from build123d import *

# Parameters (mm, degrees)
SKETCH1_R                    = 3
SKETCH1_R_2                  = 4
BASE_FLANGE1_DEPTH           = 2
SKETCH6_W                    = 90.588867986
SKETCH6_H                    = 42.612496281
CUT_EXTRUDE1_DEPTH           = 10
DELETEFACE2_START            = -2
DELETEFACE2_DEPTH            = 2
DELETEFACE3_START            = 50
DELETEFACE3_OUTLINE_W        = 40
DELETEFACE3_OUTLINE_H        = 2
DELETEFACE3_DEPTH            = 10
EDGE_FLANGE1_STRIP_W         = 9.4732
EDGE_FLANGE1_STRIP_H         = 2
EDGE_FLANGE1_STRIP_CUT_DEPTH = 40
EDGE_FLANGE1_DEPTH           = 40
EDGE_FLANGE2_STRIP_W         = 9.4732
EDGE_FLANGE2_STRIP_H         = 2
EDGE_FLANGE2_STRIP_CUT_DEPTH = 40
EDGE_FLANGE2_DEPTH           = 40
SKETCH15_R                   = 2.5
CUT_EXTRUDE2_DEPTH           = 10
CHAMFER1_SIZE                = 5
FILLET1_R                    = 5


# Read off the part's stored shape, not the designer's step: DeleteFace2, DeleteFace3
# Sheet-metal steps are written as plain solids
with BuildPart() as part:
    # Sketch1 → Base-Flange1 (new body)
    with BuildSketch(Plane(origin=(0, 0, 0), x_dir=(1, 0, 0), z_dir=(0, 1, 0))):
        with BuildLine():
            Line((-17.071067812, 52.928932188), (-12.928932188, 57.071067812))
            ThreePointArc((-12.928932188, 57.071067812), (-9.6846987, 59.238795325), (-5.857864376, 60))
            Line((-5.857864376, 60), (5.857864376, 60))
            ThreePointArc((5.857864376, 60), (9.6846987, 59.238795325), (12.928932188, 57.071067812))
            Line((12.928932188, 57.071067812), (17.071067812, 52.928932188))
            ThreePointArc((17.071067812, 52.928932188), (19.238795325, 49.6846987), (20, 45.857864376))
            Line((20, 45.857864376), (20, -45.857864376))
            ThreePointArc((20, -45.857864376), (19.238795325, -49.6846987), (17.071067812, -52.928932188))
            Line((17.071067812, -52.928932188), (12.928932188, -57.071067812))
            ThreePointArc((12.928932188, -57.071067812), (9.6846987, -59.238795325), (5.857864376, -60))
            Line((5.857864376, -60), (-5.857864376, -60))
            ThreePointArc((-5.857864376, -60), (-9.6846987, -59.238795325), (-12.928932188, -57.071067812))
            Line((-12.928932188, -57.071067812), (-17.071067812, -52.928932188))
            ThreePointArc((-17.071067812, -52.928932188), (-19.238795325, -49.6846987), (-20, -45.857864376))
            Line((-20, -45.857864376), (-20, -39.142135624))
            ThreePointArc((-20, -39.142135624), (-20.761204675, -35.3153013), (-22.928932188, -32.071067812))
            Line((-22.928932188, -32.071067812), (-27.071067812, -27.928932188))
            ThreePointArc((-27.071067812, -27.928932188), (-30.3153013, -25.761204675), (-34.142135624, -25))
            Line((-34.142135624, -25), (-45.857864376, -25))
            ThreePointArc((-45.857864376, -25), (-49.6846987, -24.238795325), (-52.928932188, -22.071067812))
            Line((-52.928932188, -22.071067812), (-57.071067812, -17.928932188))
            ThreePointArc((-57.071067812, -17.928932188), (-59.238795325, -14.6846987), (-60, -10.857864376))
            Line((-60, -10.857864376), (-60, 10.857864376))
            ThreePointArc((-60, 10.857864376), (-59.238795325, 14.6846987), (-57.071067812, 17.928932188))
            Line((-57.071067812, 17.928932188), (-52.928932188, 22.071067812))
            ThreePointArc((-52.928932188, 22.071067812), (-49.6846987, 24.238795325), (-45.857864376, 25))
            Line((-45.857864376, 25), (-34.142135624, 25))
            ThreePointArc((-34.142135624, 25), (-30.3153013, 25.761204675), (-27.071067812, 27.928932188))
            Line((-27.071067812, 27.928932188), (-22.928932188, 32.071067812))
            ThreePointArc((-22.928932188, 32.071067812), (-20.761204675, 35.3153013), (-20, 39.142135624))
            Line((-20, 39.142135624), (-20, 45.857864376))
            ThreePointArc((-20, 45.857864376), (-19.238795325, 49.6846987), (-17.071067812, 52.928932188))
        make_face()
        with Locations(Location((0, 42.5, 0), (0, 0, 270))):
            Circle(SKETCH1_R, mode=Mode.SUBTRACT)
        with Locations(Location((0, -42.5, 0), (0, 0, 270))):
            Circle(SKETCH1_R, mode=Mode.SUBTRACT)
        with Locations(Location((0, 0, 0), (0, 0, 270))):
            Circle(SKETCH1_R_2, mode=Mode.SUBTRACT)
        with Locations(Location((-35.23885867, -15, 0), (0, 0, 270))):
            Circle(SKETCH1_R_2, mode=Mode.SUBTRACT)
        with Locations(Location((-35.23885867, 15, 0), (0, 0, 270))):
            Circle(SKETCH1_R_2, mode=Mode.SUBTRACT)
    extrude(amount=-BASE_FLANGE1_DEPTH)

    # Sketch6 → Cut-Extrude1 (cut)
    with BuildSketch(Plane(origin=(0, 0, 0), x_dir=(1, 0, 0), z_dir=(0, 1, 0))):
        with Locations((11.152298369, 46.306248141)):
            Rectangle(SKETCH6_W, SKETCH6_H)
    extrude(amount=-CUT_EXTRUDE1_DEPTH, mode=Mode.SUBTRACT)

    # DeleteFace2 outline → DeleteFace2 (add)
    with BuildSketch(Plane(origin=(0, 0, 0), x_dir=(1, 0, 0), z_dir=(0, 1, 0)).offset(DELETEFACE2_START)):
        with BuildLine():
            Line((5.857864376, -60), (10, -60))
            Line((10, -60), (12.928932188, -57.071067812))
            ThreePointArc((12.928932188, -57.071067812), (9.6846987, -59.238795325), (5.857864376, -60))
        make_face()
        with BuildLine():
            Line((-20, -50), (-17.071067812, -52.928932188))
            ThreePointArc((-17.071067812, -52.928932188), (-19.238795325, -49.6846987), (-20, -45.857864376))
            Line((-20, -45.857864376), (-20, -50))
        make_face()
        with BuildLine():
            Line((-10, -60), (-5.857864376, -60))
            ThreePointArc((-5.857864376, -60), (-9.6846987, -59.238795325), (-12.928932188, -57.071067812))
            Line((-12.928932188, -57.071067812), (-10, -60))
        make_face()
        with BuildLine():
            ThreePointArc((20, -45.857864376), (19.238795325, -49.6846987), (17.071067812, -52.928932188))
            Line((17.071067812, -52.928932188), (20, -50))
            Line((20, -50), (20, -45.857864376))
        make_face()
    extrude(amount=DELETEFACE2_DEPTH)

    # DeleteFace3 outline → DeleteFace3 (add)
    with BuildSketch(Plane.XY.offset(DELETEFACE3_START)):
        with Locations((0, -1)):
            Rectangle(DELETEFACE3_OUTLINE_W, DELETEFACE3_OUTLINE_H)
    extrude(amount=DELETEFACE3_DEPTH)

    # Edge-Flange1 strip (across the edge) → Edge-Flange1 strip cut (cut)
    with BuildSketch(Plane(origin=(-20, 0, 60), x_dir=(0, 0, -1), z_dir=(1, 0, 0))):
        with Locations((-2, -1)):
            Rectangle(EDGE_FLANGE1_STRIP_W, EDGE_FLANGE1_STRIP_H)
    extrude(amount=EDGE_FLANGE1_STRIP_CUT_DEPTH, mode=Mode.SUBTRACT)

    # Edge-Flange1 section (across the edge) → Edge-Flange1 (add)
    with BuildSketch(Plane(origin=(-20, 0, 60), x_dir=(0, 0, -1), z_dir=(1, 0, 0))):
        with BuildLine():
            Line((0, 0.7366), (0, 48))
            Line((0, 48), (2, 48))
            Line((2, 48), (2, 0.7366))
            ThreePointArc((2, 0.7366), (2.215745145, 0.215745145), (2.7366, 0))
            Line((2.7366, 0), (2.7366, -2))
            ThreePointArc((2.7366, -2), (0.801531583, -1.198468417), (0, 0.7366))
        make_face()
    extrude(amount=EDGE_FLANGE1_DEPTH)

    # Edge-Flange2 strip (across the edge) → Edge-Flange2 strip cut (cut)
    with BuildSketch(Plane(origin=(-20, 48, 58), x_dir=(0, -1, 0), z_dir=(1, 0, 0))):
        with Locations((-2, -1)):
            Rectangle(EDGE_FLANGE2_STRIP_W, EDGE_FLANGE2_STRIP_H)
    extrude(amount=EDGE_FLANGE2_STRIP_CUT_DEPTH, mode=Mode.SUBTRACT)

    # Edge-Flange2 section (across the edge) → Edge-Flange2 (add)
    with BuildSketch(Plane(origin=(-20, 48, 58), x_dir=(0, -1, 0), z_dir=(1, 0, 0))):
        with BuildLine():
            Line((0, 0.7366), (0, 58))
            Line((0, 58), (2, 58))
            Line((2, 58), (2, 0.7366))
            ThreePointArc((2, 0.7366), (2.215745145, 0.215745145), (2.7366, 0))
            Line((2.7366, 0), (2.7366, -2))
            ThreePointArc((2.7366, -2), (0.801531583, -1.198468417), (0, 0.7366))
        make_face()
    extrude(amount=EDGE_FLANGE2_DEPTH)

    # Sketch15 → Cut-Extrude2 (cut)
    with BuildSketch(Plane(origin=(0, 48, 0), x_dir=(1, 0, 0), z_dir=(0, 1, 0))):
        with Locations(Location((-12, -8, 0), (0, 0, 270))):
            Circle(SKETCH15_R)
        with Locations(Location((12, -8, 0), (0, 0, 270))):
            Circle(SKETCH15_R)
    extrude(amount=-CUT_EXTRUDE2_DEPTH, mode=Mode.SUBTRACT)

    # Chamfer1
    chamfer1_edges = [part.edges().sort_by_distance(p)[0] for p in [
        (20, -1, -25),
        (-20, 47, 0),
        (20, 47, 0),
    ]]
    chamfer(chamfer1_edges, length=CHAMFER1_SIZE)

    # Fillet1
    fillet1_edges = [part.edges().sort_by_distance(p)[0] for p in [
        (15, -1, -25),
        (20, -1, -20),
        (-15, 47, 0),
        (15, 47, 0),
        (20, 47, 5),
        (-20, 47, 5),
    ]]
    fillet(fillet1_edges, radius=FILLET1_R)


solid = part.part
Source: CAD feature listing. Evaluate the final solid. Frame: model axes, mm. A direction names the side the tool comes from. Coordinates: 2 decimals unless noted, no trailing zeros. Loops run counter-clockwise (first coordinate to the right, second up) from the corner with the lowest first, then second, coordinate; pieces in that order, holes last. Notation, with made-up numbers: (62.25, 48) - (89.25, 48) arc R22 cw to (89.25, 77) - close; hole circle Ø9 at (-10.75, -11). An arc over 180 degrees is marked (long way). One line per item, written item: value. Start each with the question number.
1. Contact query for flat-ended pins moving along their axis: P1, Ø1.6, axis at x = -37, y = -1.5, coming from the +Z side; P2, Ø1, axis at x = 12, y = 8.5, coming from the -Z side; P3, Ø1, axis at x = -13.5, z = -13, coming from the +Y side; P4, Ø7, axis at x = -35.24, z = 15, coming from the +Y side. Output: stop coordinate, or through.
2. Section A-A (x = 0). Return the cut outline in (y, z), and give its area (3 significant figures).
3. Section D-D (y = 21). Return the cut outline in (x, z).
4. Mould query, pull axis X, two halves, no side actions, for faces 5 (the cylindrical face through (-30.265, -0.986, 25.782)), 6 (the flat face through (20, 19.2, 58.4)), 7 (the cylindrical face through (0.1, -1, 39.5)). Classes: pulls with the +X half, pulls with the -X half, needs draft (parallel to the pull), parting line crosses it, or undercut.
5. Set-up query: faces 1 (the flat face through (0, 48, 29)), 2 (the cylindrical face through (9.78, 47.01, 9.15)), 3 (the flat face through (17, 47, 2)), 4 (the flat face through (-17, 47, 2)). Return all of +Z, -Z, +X, -X, +Y, -Y with unobstructed straight access to the full face (end or side cutting, diameter ignored); none if empty.
6. Section B-B (z = 42.5). Return the cut outline in (x, y).
7. Ray query, L1, parallel to X at y = 47.4, z = 8; L2, parallel to Y at x = 7, z = 35; L3, parallel to X at y = -1.4, z = 42.5. Return the intervals inside material, ascending.
8. Section C-C (z = -15). Return the cut outline in (x, y).
Verdict:
1. P1: stops at z = 25
1. P2: stops at z = 58
1. P3: stops at y = 0
1. P4: passes through
2. outline: (-2, -25) - (0, -25) - (0, -4) - (-2, -4) - close; (-2, 4) - (0, 4) - (0, 39.5) - (-2, 39.5) - close; (-2, 45.5) - (0, 45.5) - (0, 57.26) arc R0.74 cw to (0.74, 58) - (45.26, 58) arc R0.74 cw to (46, 57.26) - (46, 0) - (48, 0) - (48, 57.26) arc R2.74 ccw to (45.26, 60) - (0.74, 60) arc R2.74 ccw to (-2, 57.26) - close
2. area: 351 mm2
3. outline: (-20, 58) - (20, 58) - (20, 60) - (-20, 60) - close
4. face 5: pulls with the -X half
4. face 6: pulls with the +X half
4. face 7: undercut
5. face 1: +Z, -Z, +X, -X, +Y
5. face 2: +Y
5. face 3: -Z, +X, +Y
5. face 4: -Z, -X, +Y
6. outline: (-20, -2) - (-3, -2) - (-3, 0) - (-20, 0) - close; (-20, 46) - (20, 46) - (20, 48) - (-20, 48) - close; (3, -2) - (20, -2) - (20, 0) - (3, 0) - close
7. L1: x = -20 to -14.5, -9.5 to 9.5, 14.5 to 20
7. L2: y = -2 to 0, 46 to 48
7. L3: x = -20 to -3, 3 to 20
8. outline: (-59.1, -2) - (-39.24, -2) - (-39.24, 0) - (-59.1, 0) - close; (-31.24, -2) - (20, -2) - (20, 0) - (-31.24, 0) - close
